from build123d import *

# Parameters (mm, degrees)
SKETCH1_R          = 3.175
EXTRUDE1_DEPTH     = 38.1
SKETCH6_R          = 4.7625
EXTRUDE2_DEPTH     = 6.35
CUT_EXTRUDE1_DEPTH = 3.571875
SKETCH8_R          = 2.749630657
CUT_EXTRUDE2_DEPTH = 0.635
CUT_EXTRUDE2_DRAFT = -45
CHAMFER1_SIZE      = 0.635
CHAMFER2_SIZE      = 0.3175
CHAMFER3_SIZE      = 0.9525


with BuildPart() as part:
    # Sketch1 → Extrude1 (new body)
    with BuildSketch(Plane.XY):
        Circle(SKETCH1_R)
    extrude(amount=-EXTRUDE1_DEPTH)

    # Sketch6 → Extrude2 (add)
    with BuildSketch(Plane(origin=(0, 0, -38.1), x_dir=(-1, 0, 0), z_dir=(0, 0, -1))):
        Circle(SKETCH6_R)
    extrude(amount=EXTRUDE2_DEPTH)

    # Sketch7 → Cut-Extrude1 (cut)
    with BuildSketch(Plane(origin=(0, 0, -44.45), x_dir=(-1, 0, 0), z_dir=(0, 0, -1))):
        Polygon((0, 2.749630657), (-2.38125, 1.374815329), (-2.38125, -1.374815329), (0, -2.749630657), (2.38125, -1.374815329), (2.38125, 1.374815329), align=None)
    extrude(amount=-CUT_EXTRUDE1_DEPTH, mode=Mode.SUBTRACT)


with BuildPart() as cut_extrude2_tool:
    # Sketch8 → Cut-Extrude2 (with draft: the straight prism first)
    with BuildSketch(Plane(origin=(0, 0, -44.45), x_dir=(-1, 0, 0), z_dir=(0, 0, -1))):
        Circle(SKETCH8_R)
    extrude(amount=-CUT_EXTRUDE2_DEPTH)
    # Cut-Extrude2: the draft: its side faces are tilted about the plane it starts from
    cut_extrude2_sides = [cut_extrude2_tool.faces().sort_by_distance(p)[0] for p in [
        (2.749630657, 0, -44.1325),
    ]]
    draft(cut_extrude2_sides, Plane(origin=(0, 0, -44.45), x_dir=(-1, 0, 0), z_dir=(0, 0, -1)), CUT_EXTRUDE2_DRAFT)


with BuildPart() as part_1:
    add(part.part)

    # Cut-Extrude2: cut by cut_extrude2_tool
    add(cut_extrude2_tool.part, mode=Mode.SUBTRACT)

    # Chamfer1
    chamfer1_edges = [part_1.edges().sort_by_distance(p)[0] for p in [
        (4.7625, 0, -44.45),
    ]]
    chamfer(chamfer1_edges, length=CHAMFER1_SIZE)

    # Chamfer2
    chamfer2_edges = [part_1.edges().sort_by_distance(p)[0] for p in [
        (4.7625, 0, -38.1),
    ]]
    chamfer(chamfer2_edges, length=CHAMFER2_SIZE)

    # Chamfer3
    chamfer3_edges = [part_1.edges().sort_by_distance(p)[0] for p in [
        (-3.175, 0, 0),
    ]]
    chamfer(chamfer3_edges, length=CHAMFER3_SIZE)


solid = part_1.part
CAD build for the part. Positions are in the model's coordinates, mm. A direction names the side the tool comes from. Give positions to 0.01 mm unless a question says otherwise; leave off trailing zeros. Write each loop counter-clockwise with the first axis right and the second up, starting at its lowest first coordinate (ties: lowest second). Pieces come first, ordered by that corner, then holes. Notation, with made-up numbers: (36.5, -7.75) - (69.5, -7.75) arc R23 ccw to (69.5, 4.25) - close; hole circle Ø8 at (-6.5, -11). An arc over 180 degrees is marked (long way). Put each result on its own line as item: value.
(1) Tool access for faces 4 (the cylindrical face through (3.78, -2.9, -41.08)), 5 (the conical face through (-1.268, -2.233, -44.268)): list every direction of +Z, -Z, +X, -X, +Y, -Y with a clear straight run to the whole face (end or side of a thin tool).
Working result:
face 4: +Z, -Z
face 5: -Z
(2) Drop flat-ended pins along their axis: pin 1 Ø4 at (x, z) = (-1, -27) entering from +Y (3 decimals); pin 2 Ø1.5 at (y, z) = (2.5, -28.5) entering from +X. Give the stop position or say it passes through.
Working result:
pin 1: y = 3.175
pin 2: x = 2.65
(3) Pull direction X, two halves, no side cores. Call faces 1 (the cylindrical face through (-0.69, -3.1, -19.27)), 2 (the flat face through (-2, -3, -38.1)), 3 (the flat face through (-2.381, 0, -43)): released by +X, released by -X, zero draft, split by the parting line, or undercut.
Working result:
face 1: split by the parting line
face 2: zero draft
face 3: undercut
(4) Wall check: L1, parallel to Y at x = -0.25, z = -6.5; L2, parallel to X at y = 1.5, z = -41.5; L3, parallel to Z at x = -1.25, y = -3. Give the ranges that are in metal, low to high.
Working result:
L1: -3.17 to 3.17
L2: -4.52 to -2.16, 2.16 to 4.52
L3: -44.45 to -38.1
(5) Saw through at B-B (z = -40.5). List the corners of the cut face in (x, y) (1 decimal).
Working result:
outline: circle Ø9.5 at (0, 0)
(6) Saw through at C-C (z = -11). List the corners of the cut face in (x, y) (3 decimals).
Working result:
outline: circle Ø6.35 at (0, 0)
